from build123d import *

# Parameters (mm, degrees)
CROQUIS1_W                       = 10
CROQUIS1_H                       = 15
BRIDA_BASE1_DEPTH                = 0.7366
BRIDA_DE_ARISTA1_STRIP_W         = 4.4196
BRIDA_DE_ARISTA1_STRIP_H         = 0.7366
BRIDA_DE_ARISTA1_STRIP_CUT_DEPTH = 10
BRIDA_DE_ARISTA1_DEPTH           = 10
CROQUIS7_R                       = 1.5
CORTAR_EXTRUIR1_DEPTH            = 10


# Sheet-metal steps are written as plain solids
with BuildPart() as part:
    # Croquis1 → Brida base1 (new body)
    with BuildSketch(Plane(origin=(0, 0, 0), x_dir=(1, 0, 0), z_dir=(0, 1, 0))):
        Rectangle(CROQUIS1_W, CROQUIS1_H)
    extrude(amount=-BRIDA_BASE1_DEPTH)

    # Brida de arista1 strip (across the edge) → Brida de arista1 strip cut (cut)
    with BuildSketch(Plane(origin=(-5, 0, 7.5), x_dir=(0, 0, -1), z_dir=(1, 0, 0))):
        with Locations((-1.4732, -0.3683)):
            Rectangle(BRIDA_DE_ARISTA1_STRIP_W, BRIDA_DE_ARISTA1_STRIP_H)
    extrude(amount=BRIDA_DE_ARISTA1_STRIP_CUT_DEPTH, mode=Mode.SUBTRACT)

    # Brida de arista1 section (across the edge) → Brida de arista1 (add)
    with BuildSketch(Plane(origin=(-5, 0, 7.5), x_dir=(0, 0, -1), z_dir=(1, 0, 0))):
        with BuildLine():
            Line((-0.7366, 0.7366), (-0.7366, 10))
            Line((-0.7366, 10), (0, 10))
            Line((0, 10), (0, 0.7366))
            ThreePointArc((0, 0.7366), (0.215745145, 0.215745145), (0.7366, 0))
            Line((0.7366, 0), (0.7366, -0.7366))
            ThreePointArc((0.7366, -0.7366), (-0.30510971, -0.30510971), (-0.7366, 0.7366))
        make_face()
    extrude(amount=BRIDA_DE_ARISTA1_DEPTH)

    # Croquis7 → Cortar-Extruir1 (cut)
    with BuildSketch(Plane.XY.offset(8.2366)):
        with Locations((0, 7)):
            Circle(CROQUIS7_R)
    extrude(amount=-CORTAR_EXTRUIR1_DEPTH, mode=Mode.SUBTRACT)


solid = part.part
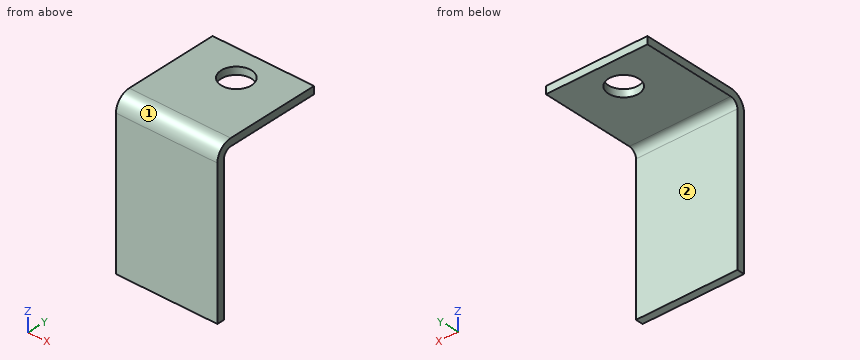
The listing builds one solid part. Answer for the finished solid, in the listing's coordinates (mm). Face numbers are marked on the shaded views. A direction names the side the tool comes from. Round coordinates to 2 decimals unless told otherwise and drop trailing zeros. Order: outer loops, then holes, each group sorted by start corner. A loop starts at its lowest first (then second) coordinate and runs counter-clockwise, first axis right, second up. Notation, with made-up numbers: M -32,76 L -13,76 A32 ccw -13,105 Z; hole C 41,37 d7. An arc over 180 degrees is marked long. Answer in a Markdown table with one row per item. Add a question column.
1) Which of the six approach directions +Z, -Z, +X, -X, +Y, -Y give full straight-line access (tool end or side, diameter ignored) to the marked faces 1 and 2?
2) Flat-ended cylindrical pins translate along their axes: pin 1 Ø4 at (y, z) = (2.5, -4) entering from +X; pin 2 Ø4 at (x, z) = (-0.5, -5.5) entering from +Y; pin 3 Ø2 at (x, y) = (2.5, 6) entering from -Z. Find the tip coordinate at first contact, or state that the pin passes through.
3) The part is cut by section A-A on y = 7. Determine the outline of the cut face in (x, z).
4) The part is cut by section C-C on x = 3. Determine the outline of the cut face in (y, z), plus the area to 3 significant figures.
5) Consider line 1 along Y through (x, z) = (-0.75, 5); line 2 along Z through (x, y) = (3.75, 9.25); line 3 along Y through (x, z) = (0, 8.05). Determine where each line is inside the solid, lowest interval first. Write a range as from..to.
6) The part is cut by section D-D on y = 3.75. Determine the outline of the cut face in (x, z), plus the area to 3 significant figures.
7) The part is cut by section B-B on x = 0. Determine the outline of the cut face in (y, z), plus the area to 3 significant figures.
Findings below:
| question | item | result |
|---|---|---|
| 1 | face 1 | +Z, +X, -X, -Y |
| 1 | face 2 | -Z, +X, -X, +Y |
| 2 | pin 1 | passes through |
| 2 | pin 2 | stops at y = 0 |
| 2 | pin 3 | stops at z = 7.5 |
| 3 | outline | M -5,7.5 L -1.5,7.5 L -1.5,8.24 L -5,8.24 Z; M 1.5,7.5 L 5,7.5 L 5,8.24 L 1.5,8.24 Z |
| 4 | outline | M -0.74,-7.5 L 0,-7.5 L 0,6.76 A0.74 cw 0.74,7.5 L 10,7.5 L 10,8.24 L 0.74,8.24 A1.47 ccw -0.74,6.76 Z |
| 4 | area | 18.6 mm² |
| 5 | line 1 | y = -0.74..0 |
| 5 | line 2 | z = 7.5..8.24 |
| 5 | line 3 | y = 0.02..5.5, 8.5..10 |
| 6 | outline | M -5,7.5 L 5,7.5 L 5,8.24 L -5,8.24 Z |
| 6 | area | 7.37 mm² |
| 7 | outline | M -0.74,-7.5 L 0,-7.5 L 0,6.76 A0.74 cw 0.74,7.5 L 5.5,7.5 L 5.5,8.24 L 0.74,8.24 A1.47 ccw -0.74,6.76 Z; M 8.5,7.5 L 10,7.5 L 10,8.24 L 8.5,8.24 Z |
| 7 | area | 16.4 mm² |
